```python
from build123d import *

# Parameters (mm, degrees)
SKETCH1_R           = 27.5
BOSS_EXTRUDE1_DEPTH = 3
SKETCH2_R           = 1.25
CUT_EXTRUDE1_DEPTH  = 3
CUT_EXTRUDE5_START  = -3
SKETCH3_R           = 5
SKETCH3_R_2         = 1.25
CUT_EXTRUDE5_DEPTH  = 3


with BuildPart() as part:
    # Sketch1 → Boss-Extrude1 (new body)
    with BuildSketch(Plane(origin=(0, 0, 0), x_dir=(1, 0, 0), z_dir=(0, 1, 0))):
        with Locations(Location((0, 0, 0), (0, 0, 270))):
            Circle(SKETCH1_R)
    extrude(amount=BOSS_EXTRUDE1_DEPTH)

    # Sketch2 → Cut-Extrude1 (cut)
    with BuildSketch(Plane(origin=(0, 3, 0), x_dir=(1, 0, 0), z_dir=(0, 1, 0))):
        with Locations(Location((0, -25, 0), (0, 0, 270))):
            Circle(SKETCH2_R)
        with Locations(Location((24, 7, 0), (0, 0, 270))):
            Circle(SKETCH2_R)
        with Locations(Location((-19, 16.248076809, 0), (0, 0, 270))):
            Circle(SKETCH2_R)
    extrude(amount=-CUT_EXTRUDE1_DEPTH, mode=Mode.SUBTRACT)

    # Sketch3 → Cut-Extrude5 (cut)
    with BuildSketch(Plane(origin=(0, 3, 0), x_dir=(1, 0, 0), z_dir=(0, 1, 0)).offset(CUT_EXTRUDE5_START)):
        with BuildLine():
            Line((-2.196984727, -5.970983825), (22.703158369, 9.137335206))
            ThreePointArc((22.703158369, 9.137335206), (24.905937464, 9.330080967), (26.399999989, 7.700000036))
            ThreePointArc((26.399999989, 7.700000036), (5.782248195, 26.885230254), (-20.900000036, 17.872884448))
            ThreePointArc((-20.900000036, 17.872884448), (-18.646279407, 18.722926652), (-16.720914968, 17.275584191))
            Line((-16.720914968, 17.275584191), (-6.898195472, -4.511911817))
            ThreePointArc((-6.898195472, -4.511911817), (-4.415107472, -4.814581464), (-2.196984727, -5.970983825))
        make_face()
        with BuildLine():
            ThreePointArc((26.5, 7), (26.178543559, 5.773644439), (25.296841631, 4.862664794))
            Line((25.296841631, 4.862664794), (0.396698535, -10.245654238))
            ThreePointArc((0.396698535, -10.245654238), (0.481617092, -10.870273767), (0.51, -11.5))
            ThreePointArc((0.51, -11.5), (0.013935278, -14.088209014), (-1.403950257, -16.309583974))
            Line((-1.403950257, -16.309583974), (2.253156128, -23.916816054))
            ThreePointArc((2.253156128, -23.916816054), (2.437507982, -24.444522872), (2.5, -25))
            ThreePointArc((2.5, -25), (1.767766953, -26.767766953), (0, -27.5))
            ThreePointArc((0, -27.5), (19.445436483, -19.445436483), (27.5, 0))
            ThreePointArc((27.5, 0), (27.223611073, 3.889087315), (26.399999989, 7.700000036))
            ThreePointArc((26.399999989, 7.700000036), (26.474873731, 7.353553409), (26.5, 7))
        make_face()
        with Locations(Location((-6.49, -11.5, 0), (0, 0, 270))):
            Circle(SKETCH3_R)
        with Locations(Location((0, -25, 0), (0, 0, 270))):
            Circle(SKETCH3_R_2)
        with Locations(Location((24, 7, 0), (0, 0, 270))):
            Circle(SKETCH3_R_2)
        with Locations(Location((-19, 16.248076809, 0), (0, 0, 270))):
            Circle(SKETCH3_R_2)
        with BuildLine():
            ThreePointArc((-21.279085032, 15.220569428), (-21.474849842, 16.601797402), (-20.900000036, 17.872884448))
            ThreePointArc((-20.900000036, 17.872884448), (-24.977533128, -11.505339579), (0, -27.5))
            ThreePointArc((0, -27.5), (-1.330796779, -27.116360067), (-2.253156128, -26.083183946))
            Line((-2.253156128, -26.083183946), (-5.910262513, -18.475951867))
            ThreePointArc((-5.910262513, -18.475951867), (-12.835616379, -14.455190818), (-11.456365535, -6.56692658))
            Line((-11.456365535, -6.56692658), (-21.279085032, 15.220569428))
        make_face()
    extrude(amount=CUT_EXTRUDE5_DEPTH, mode=Mode.SUBTRACT)


solid = part.part
```
Could you check a few things on this model? Use its own coordinates, in mm. A direction names the side the tool comes from. Give positions to 0.01 mm unless a question says otherwise; leave off trailing zeros. Order: outer loops, then holes, each group sorted by start corner. A loop starts at its lowest first (then second) coordinate and runs counter-clockwise, first axis right, second up.
Q1. Suppose I cut it at D-D, the plane x = 12. Write out the boundary of the cut face in (y, z), and give its area (3 significant figures).
Q2. We'd pull the mould along X, two halves only. Please class faces 1 (the flat face through (-16.299, 1.479, -4.174)), 2 (the flat face through (-3, 3, 6)), 3 (the flat face through (13, 1.5, 2.6)), 4 (the flat face through (10.08, 1.48, -1.48)): +X half, -X half, draft (parallel to the pull), parting line (faces both ways), or undercut.
Q3. Suppose I cut it at B-B, the plane z = -3.5. Write out the boundary of the cut face in (x, y), and give its area (3 significant figures).
Q4. If I drill on line 1 along X through (y, z) = (0.6, 11.5); line 2 along X through (y, z) = (1.95, 1); line 3 along Z through (x, y) = (23.5, 1.15), over which ranges is the centre line in solid material (lowest first)?
Q5. For faces 5 (the flat face through (0.4, 1.48, 20.06)), 6 (the cylindrical face through (-4.99, 1.48, 16.27)), 7 (the cylindrical face through (-4.449, 1.479, 4.804)), which set-ups out of +Z, -Z, +X, -X, +Y, -Y let a thin tool reach every point of the face, with its end or its side?
Q6. Suppose I cut it at A-A, the plane y = 2.45. Write out the boundary of the cut face in (x, z).
Q7. Suppose I cut it at C-C, the plane x = -10. Write out the boundary of the cut face in (y, z).
Q8. I'm going to push flat-ended pins straight in: P1, Ø3, axis at x = 24, z = -7, coming from the -Y side; P2, Ø2, axis at x = -19, z = -16.25, coming from the +Y side; P3, Ø1, axis at y = 2, z = 13, coming from the +X side; P4, Ø1.5, axis at x = 1, y = 1.5, coming from the -Z side. Where does each tip first touch, or does it pass through?
Solution:
1. outline: (0, -2.64) - (3, -2.64) - (3, 3.21) - (0, 3.21) - close
1. area: 17.5 mm2
2. face 1: -X half
2. face 2: draft
2. face 3: +X half
2. face 4: undercut
3. outline: (-15.99, 0) - (-10.51, 0) - (-10.51, 3) - (-15.99, 3) - close; (13.41, 0) - (23.05, 0) - (23.05, 3) - (13.41, 3) - close
3. area: 45.4 mm2
4. line 1: x = -13.49 to -11.49, -1.49 to 0.51
4. line 2: x = -13.97 to -8.48, 6 to 15.63
4. line 3: z = -9.45 to -8.15, -5.85 to -3.77
5. face 5: +X, +Y, -Y
5. face 6: +Y, -Y
5. face 7: -Z, +Y, -Y
6. outline: (-21.28, -15.22) arc R2.5 ccw to (-16.72, -17.28) - (-6.9, 4.51) arc R7 ccw to (-2.2, 5.97) - (22.7, -9.14) arc R2.5 ccw to (25.3, -4.86) - (0.4, 10.25) arc R7 ccw to (-1.4, 16.31) - (2.25, 23.92) arc R2.5 ccw to (-2.25, 26.08) - (-5.91, 18.48) arc R7 ccw to (-11.46, 6.57) - close; hole circle Ø2.5 at (-19, -16.25); hole circle Ø10 at (-6.49, 11.5); hole circle Ø2.5 at (0, 25); hole circle Ø2.5 at (24, -7)
7. outline: (0, -2.37) - (3, -2.37) - (3, 7.94) - (0, 7.94) - close; (0, 15.06) - (3, 15.06) - (3, 17.56) - (0, 17.56) - close
8. P1: stops at y = 0
8. P2: passes through
8. P3: stops at x = 0.44
8. P4: stops at z = 3.58
